```python
from build123d import *

# Parameters (mm, degrees)
SKETCH1_R           = 1.75
BOSS_EXTRUDE1_DEPTH = 8
FILLET1_R           = 10


with BuildPart() as part:
    # Sketch1 → Boss-Extrude1 (new body)
    with BuildSketch(Plane.XY):
        with BuildLine():
            Line((0, 0), (-2, 0))
            Line((-2, 0), (-2, 4))
            Line((-2, 4), (11, 4))
            ThreePointArc((11, 4), (12.171572875, 6.828427125), (15, 8))
            Line((15, 8), (15, 54))
            Line((15, 54), (18, 54))
            Line((18, 54), (18, 6.645751311))
            ThreePointArc((18, 6.645751311), (17.828427125, 1.171572875), (12.354248689, 1))
            Line((12.354248689, 1), (0, 1))
            Line((0, 1), (0, 0))
        make_face()
        with Locations((15, 4)):
            Circle(SKETCH1_R, mode=Mode.SUBTRACT)
    extrude(amount=BOSS_EXTRUDE1_DEPTH)

    # Fillet1
    # the kernel refuses this fillet: 10 mm, written as the material it adds along each edge
    with BuildSketch(Plane(origin=(11, 4, 0), x_dir=(-1, 0, 0), z_dir=(0, 0, 1))) as fillet1_piece_1:
        with BuildLine():
            CenterArc((5.797958971, -10), FILLET1_R, 90, 44.415308597)
            ThreePointArc((-1.200583151, -2.857142857), (-0.31234035, -1.549569715), (0, 0))
            Line((0, 0), (5.797958971, 0))
        make_face()
    extrude(amount=8)
    with BuildSketch(Plane(origin=(15, 8, 0), x_dir=(-0.9219149126204016, -0.3873924287955524, 0), z_dir=(0, 0, 1))) as fillet1_piece_2:
        with BuildLine():
            CenterArc((6.973063718, -9.219149126), FILLET1_R, 112.792345701, 44.415308597)
            Line((-2.246085408, -5.345224838), (0, 0))
            ThreePointArc((0, 0), (1.549569715, -0.31234035), (3.09913943, 0))
        make_face()
    extrude(amount=8)
    with BuildSketch(Plane(origin=(18, 6.645751311, 0), x_dir=(0, 1, 0), z_dir=(0, 0, 1))) as fillet1_piece_3:
        with BuildLine():
            CenterArc((2.550401112, -10), FILLET1_R, 90, 21.786789298)
            ThreePointArc((-1.161136333, -0.714285714), (-0.54991438, -0.406973372), (0, 0))
            Line((0, 0), (2.550401112, 0))
        make_face()
    extrude(amount=8)
    with BuildSketch(Plane(origin=(12.354248689, 1, 0), x_dir=(-1, 0, 0), z_dir=(0, 0, 1))) as fillet1_piece_4:
        with BuildLine():
            CenterArc((2.550401112, 10), FILLET1_R, 248.213210702, 21.786789298)
            ThreePointArc((-1.161136333, 0.714285714), (-0.54991438, 0.406973372), (0, 0))
            Line((0, 0), (2.550401112, 0))
        make_face()
    extrude(amount=8)


solid = part.part
```
Source: CAD feature listing. Evaluate the final solid. Frame: model axes, mm. A direction names the side the tool comes from. Give positions to 0.01 mm unless a question says otherwise; leave off trailing zeros. Write each loop counter-clockwise with the first axis right and the second up, starting at its lowest first coordinate (ties: lowest second). Pieces come first, ordered by that corner, then holes. Notation, with made-up numbers: (9, 52) - (26, 52) arc R30 cw to (26, 89) - close; hole circle Ø9 at (73, -6). An arc over 180 degrees is marked (long way). One line per item, written item: value. Start each with the question number.
Q1. Section query C-C, the plane y = 39. Return the cut outline in (x, z), then the cut area to 3 significant figures.
Q2. Section query A-A, the plane z = 2.5. Return the cut outline in (x, y), then the cut area to 3 significant figures.
Q3. Draft query along X for faces 1 (the face through (15.5, 20.9, 8)), 2 (the face through (0, 0.5, 3.9)), 3 (the face through (18, 32, 4)), 4 (the face through (8.913, 4.714, 3.944)). Return one class per face: +X half, -X half, draft (parallel to the pull), parting line (faces both ways), or undercut.
Q4. Section query B-B, the plane x = 2. Return the cut outline in (y, z).
Q5. First-contact query: pin 1 Ø3.5 at (x, z) = (1, 3.5) entering from +Y; pin 2 Ø4 at (y, z) = (33, 3) entering from +X; pin 3 Ø4 at (x, z) = (2.5, 2) entering from -Y. Flat tips, straight axial feed; report the tip coordinate or a pass-through.
Q6. Set-up query: faces 5 (the face through (16, 54, 4)), 6 (the face through (5, 1, 4)), 7 (the face through (15, 34, 4)). Return all of +Z, -Z, +X, -X, +Y, -Y with unobstructed straight access to the full face (end or side cutting, diameter ignored); none if empty.
Q7. Material intervals for probe 1 along X at (y, z) = (22.5, 1.75); probe 2 along Y at (x, z) = (2, 1); probe 3 along Y at (x, z) = (-0.25, 4.25), sorted ascending. Write a range as from..to.
Answer:
1. outline: (15, 0) - (18, 0) - (18, 8) - (15, 8) - close
1. area: 24.0 mm2
2. outline: (-2, 0) - (0, 0) - (0, 1) - (9.8, 1) arc R10 cw to (13.52, 0.29) arc R4 ccw to (18.71, 5.48) arc R10 cw to (18, 9.2) - (18, 54) - (15, 54) - (15, 13.8) arc R10 cw to (12.17, 6.83) arc R10 cw to (5.2, 4) - (-2, 4) - close; hole circle Ø3.5 at (15, 4)
2. area: 231 mm2
3. face 1: draft
3. face 2: undercut
3. face 3: +X half
3. face 4: -X half
4. outline: (1, 0) - (4, 0) - (4, 8) - (1, 8) - close
5. pin 1: stops at y = 4
5. pin 2: stops at x = 18
5. pin 3: stops at y = 1
6. face 5: +Z, -Z, +X, -X, +Y
6. face 6: +Z, -Z, -Y
6. face 7: +Z, -Z, -X, +Y
7. probe 1: x = 15..18
7. probe 2: y = 1..4
7. probe 3: y = 0..4
